Verification items for the finished model (mm, model axes). A direction names the side the tool comes from. Round coordinates to 2 decimals unless told otherwise and drop trailing zeros. Write each loop counter-clockwise with the first axis right and the second up, starting at its lowest first coordinate (ties: lowest second). Pieces come first, ordered by that corner, then holes. Notation, with made-up numbers: (-19.5, 71.5) -> (-8.5, 71.5) arc R24 ccw to (-8.5, 102.5) -> close; hole circle Ø10 at (62.5, 88.25). An arc over 180 degrees is marked (long way). Use CSV: the item, a comma, the result in double quotes.
```python
from build123d import *

# Parameters (mm, degrees)
SKETCH1_W           = 115
SKETCH1_H           = 170
BOSS_EXTRUDE1_DEPTH = 7
SKETCH2_W           = 30.5
SKETCH2_H           = 29
BOSS_EXTRUDE6_DEPTH = 13
SKETCH2_6_R         = 8
BOSS_EXTRUDE9_DEPTH = 35


with BuildPart() as part:
    # Sketch1 → Boss-Extrude1 (new body)
    with BuildSketch(Plane(origin=(0, 0, 0), x_dir=(1, 0, 0), z_dir=(0, 1, 0))):
        Rectangle(SKETCH1_W, SKETCH1_H)
    extrude(amount=BOSS_EXTRUDE1_DEPTH)

    # Sketch2 → Boss-Extrude6 (add)
    with BuildSketch(Plane(origin=(0, 7, 0), x_dir=(1, 0, 0), z_dir=(0, 1, 0))):
        with Locations((-15.25, 49.5)):
            Rectangle(SKETCH2_W, SKETCH2_H)
        with Locations((15.25, 49.5)):
            Rectangle(SKETCH2_W, SKETCH2_H)
        with Locations((15.25, 9.5)):
            Rectangle(SKETCH2_W, SKETCH2_H)
        with Locations((-15.25, 9.5)):
            Rectangle(SKETCH2_W, SKETCH2_H)
        with Locations((-15.25, -30.5)):
            Rectangle(SKETCH2_W, SKETCH2_H)
        with Locations((15.25, -30.5)):
            Rectangle(SKETCH2_W, SKETCH2_H)
    extrude(amount=BOSS_EXTRUDE6_DEPTH)

    # Sketch2_6 → Boss-Extrude9 (add)
    with BuildSketch(Plane(origin=(0, 7, 0), x_dir=(1, 0, 0), z_dir=(0, 1, 0))):
        with Locations(Location((-49.5, 77, 0), (0, 0, 90))):
            Circle(SKETCH2_6_R)
        with Locations(Location((-33.4, 77, 0), (0, 0, 90))):
            Circle(SKETCH2_6_R)
        with Locations(Location((-17.3, 77, 0), (0, 0, 90))):
            Circle(SKETCH2_6_R)
        with Locations(Location((33.4, 77, 0), (0, 0, 90))):
            Circle(SKETCH2_6_R)
        with Locations(Location((49.5, 77, 0), (0, 0, 90))):
            Circle(SKETCH2_6_R)
    extrude(amount=BOSS_EXTRUDE9_DEPTH)


solid = part.part
```
Q1. Section check A-A (y = 18). Record the cut outline in (x, z).
Filled in:
outline,"circle Ø16 at (-49.5, -77); circle Ø16 at (-33.4, -77); (-30.5, -64) -> (30.5, -64) -> (30.5, -35) -> (-30.5, -35) -> close; (-30.5, -24) -> (30.5, -24) -> (30.5, 5) -> (-30.5, 5) -> close; (-30.5, 16) -> (30.5, 16) -> (30.5, 45) -> (-30.5, 45) -> close; circle Ø16 at (-17.3, -77); circle Ø16 at (33.4, -77); circle Ø16 at (49.5, -77)"
Q2. Mould release check, pull along Y, two halves, no side actions. Record for faces 5 (the flat face through (49, 42, -77)), 6 (the flat face through (-30.5, 13, 31)), 7 (the flat face through (-1, 0, -1)): released by +Y, released by -Y, zero draft, split by the parting line, or undercut.
Filled in:
face 5,"released by +Y"
face 6,"zero draft"
face 7,"released by -Y"
Q3. Access from +Z, -Z, +X, -X, +Y, -Y to the whole of each face (thin tool, end or side, straight path). Record for faces 1 (the flat face through (0, 20, -50)), 2 (the flat face through (0, 13, -64)), 3 (the flat face through (30.5, 13, -49)), 4 (the flat face through (-30.5, 13, -49)).
Filled in:
face 1,"+Z, +X, -X, +Y"
face 2,"+X, -X, +Y"
face 3,"+Z, +X, +Y"
face 4,"+Z, -X, +Y"
Q4. Section check D-D (z = 63). Record the cut outline in (x, y).
Filled in:
outline,"(-57.5, 0) -> (57.5, 0) -> (57.5, 7) -> (-57.5, 7) -> close"
Q5. Section check C-C (x = 21). Record the cut outline in (y, z).
Filled in:
outline,"(0, -85) -> (7, -85) -> (7, -64) -> (20, -64) -> (20, -35) -> (7, -35) -> (7, -24) -> (20, -24) -> (20, 5) -> (7, 5) -> (7, 16) -> (20, 16) -> (20, 45) -> (7, 45) -> (7, 85) -> (0, 85) -> close"
Q6. Go/stop test with flat-tipped pins: P1, Ø8.5, axis at x = -12, z = 37.5, coming from the +Y side; P2, Ø8, axis at x = 19, y = 25.5, coming from the -Z side; P3, Ø12, axis at y = 20.5, z = 46, coming from the -X side; P4, Ø5, axis at x = 5.5, z = 33.5, coming from the -Y side. Record where each tip stops, or that it passes through.
Filled in:
P1,"y = 20"
P2,"through"
P3,"x = -30.5"
P4,"y = 0"
Q7. Section check B-B (z = 22). Record the cut outline in (x, y), plus the area to 3 significant figures.
Filled in:
outline,"(-57.5, 0) -> (57.5, 0) -> (57.5, 7) -> (30.5, 7) -> (30.5, 20) -> (-30.5, 20) -> (-30.5, 7) -> (-57.5, 7) -> close"
area,"1,600 mm²"
Q8. Material ranges on L1, parallel to Z at x = 28.5, y = 11; L2, parallel to Z at x = -26.5, y = 10; L3, parallel to Y at x = -25, z = -53, recorded low to high.
Filled in:
L1,"-83.32 to -70.68, -64 to -35, -24 to 5, 16 to 45"
L2,"-81.05 to -72.95, -64 to -35, -24 to 5, 16 to 45"
L3,"0 to 20"
